Read the model definition and answer for the solid it produces. Units are mm, in the model's axes. Coordinates: 2 decimals unless noted, no trailing zeros. Write each loop counter-clockwise with the first axis right and the second up, starting at its lowest first coordinate (ties: lowest second). Pieces come first, ordered by that corner, then holes.
(1) Given pin 1 (1 mm diameter, centred on y = 6.5, z = 0.5, fed in from -X), flat-ended and moving along its own axis, determine where the tip first touches the part or whether it passes through.
(2) Find the intervals of material crossed by probe 1 along Y at (x, z) = (11, -4.5); probe 2 along Z at (x, y) = (16.5, -7.75); probe 3 along Z at (x, y) = (43, -7.5), in increasing order.
(3) The mould has two halves that part along Y. Classify faces 1 (the flat face through (56, 12.7, -1)), 2 (the flat face through (56, -12.7, -2)), 3 (the flat face through (114.3, 1.7, 1.5)), 4 (the flat face through (56, 0, 0)): +Y half, -Y half, draft (parallel to the pull), parting line (faces both ways), or undercut.
(4) Section B-B on y = -4 is taken. Write down the section's boundary in (x, z), then the cut area to 3 significant figures.
from build123d import *

# Parameters (mm, degrees)
BOSS_EXTRUDE1_DEPTH = 114.3
FILLET1_R           = 1.27
FILLET2_R           = 1.27


with BuildPart() as part:
    # Sketch1 → Boss-Extrude1 (new body)
    with BuildSketch(Plane(origin=(0, 0, 0), x_dir=(0, 0, -1), z_dir=(1, 0, 0))):
        Polygon((0, 8.89), (0, -8.89), (3.048, -8.89), (3.048, -6.35), (6.858, -6.35), (6.858, -12.7), (-3.81, -12.7), (-3.81, 12.7), (6.858, 12.7), (6.858, 6.35), (3.048, 6.35), (3.048, 8.89), align=None)
    extrude(amount=BOSS_EXTRUDE1_DEPTH)

    # Fillet1
    fillet1_edges = [part.edges().sort_by_distance(p)[0] for p in [
        (57.15, 8.89, 0),
        (57.15, -8.89, 0),
        (57.15, -8.89, -3.048),
        (57.15, 8.89, -3.048),
    ]]
    fillet(fillet1_edges, radius=FILLET1_R)

    # Fillet2
    fillet2_edges = [part.edges().sort_by_distance(p)[0] for p in [
        (57.15, 6.35, -3.048),
        (57.15, -6.35, -6.858),
        (57.15, 6.35, -6.858),
        (57.15, -6.35, -3.048),
        (0, 8.518025612, -2.676025612),
        (0, 6.35, -4.953),
        (0, 9.525, -6.858),
        (0, -9.525, -6.858),
        (0, -6.35, -4.953),
        (0, -8.518025612, -2.676025612),
        (0, -8.89, -1.524),
        (0, -8.518025612, -0.371974388),
        (0, 0, 0),
        (0, 8.518025612, -0.371974388),
        (0, 8.89, -1.524),
        (57.15, -12.7, -6.858),
        (0, -12.7, -1.524),
        (57.15, -12.7, 3.81),
        (0, 0, 3.81),
        (114.3, -8.518025612, -0.371974388),
        (114.3, -8.89, -1.524),
        (114.3, -8.518025612, -2.676025612),
        (114.3, -6.35, -4.953),
        (114.3, -9.525, -6.858),
        (114.3, -12.7, -1.524),
        (114.3, 0, 3.81),
        (114.3, 9.525, -6.858),
        (114.3, 6.35, -4.953),
        (114.3, 8.518025612, -2.676025612),
        (114.3, 8.89, -1.524),
        (114.3, 8.518025612, -0.371974388),
        (114.3, 0, 0),
        (57.15, 12.7, -6.858),
        (114.3, 12.7, -1.524),
        (57.15, 12.7, 3.81),
        (0, 12.7, -1.524),
    ]]
    fillet(fillet2_edges, radius=FILLET2_R - 0.0001)  # a hair under: the kernel refuses the full size


solid = part.part
Response:
1. pin 1: stops at x = 0.03
2. probe 1: y = -12.7 to -6.35, 6.35 to 12.7
2. probe 2: z = -6.86 to -3.04, -0.01 to 3.81
2. probe 3: z = -6.85 to -3.05, 0 to 3.81
3. face 1: +Y half
3. face 2: -Y half
3. face 3: draft
3. face 4: undercut
4. outline: (0, 1.27) arc R1.27 ccw to (1.27, 0) - (113.03, 0) arc R1.27 ccw to (114.3, 1.27) - (114.3, 2.54) arc R1.27 ccw to (113.03, 3.81) - (1.27, 3.81) arc R1.27 ccw to (0, 2.54) - close
4. area: 434 mm2
